The model under review builds one solid part; all positions refer to its coordinate system, in mm. A direction names the side the tool comes from. Give positions to 0.01 mm unless a question says otherwise; leave off trailing zeros. Order: outer loops, then holes, each group sorted by start corner. A loop starts at its lowest first (then second) coordinate and runs counter-clockwise, first axis right, second up. Notation, with made-up numbers: (78, -9.5) - (121, -9.5) arc R18 ccw to (121, 6.5) - close; hole circle Ø11 at (-5.75, 60.25). An arc over 180 degrees is marked (long way). Use a Markdown table: item, result. Add a question column.
```python
from build123d import *

# Parameters (mm, degrees)
RESSALTO_EXTRUS_O1_DEPTH = 25
ESBO_O2_R                = 3.75
ESBO_O2_R_2              = 1.65
CORTE_EXTRUS_O1_DEPTH    = 140.936789771
FILETE1_R                = 12.5
RESSALTO_EXTRUS_O2_REACH = 137.379
RESSALTO_EXTRUS_O3_DEPTH = 25
ESBO_O3_R                = 1.340765279
ESBO_O3_R_2              = 1.395401155
CORTE_EXTRUS_O4_DEPTH    = 25
ESBO_O10_R               = 1.55
CORTE_EXTRUS_O5_DEPTH    = 3


with BuildPart() as part:
    # Esboço1 → Ressalto-extrusão1 (new body)
    with BuildSketch(Plane(origin=(0, 0, 0), x_dir=(1, 0, 0), z_dir=(0, 1, 0))):
        Polygon((-59.715709909, 31.339816021), (-59.715709909, -1.660183979), (4.819954225, -7.306322984), (9.819954225, -7.306322984), (74.355618358, -1.660183979), (74.355618358, 31.339816021), (69.59163611, 31.339816021), (69.59163611, 2.942120769), (9.819954225, -2.287223796), (4.819954225, -2.287223796), (-54.951727661, 2.942120769), (-54.951727661, 31.339816021), align=None)
    extrude(amount=RESSALTO_EXTRUS_O1_DEPTH)

    # Esboço2 → Corte-extrusão1 (cut, through all)
    with BuildSketch(Plane(origin=(74.355618358, 0, 0), x_dir=(0, 0, -1), z_dir=(1, 0, 0))):
        with Locations((15.839816021, 12.5)):
            Circle(ESBO_O2_R)
        with Locations((24.339816021, 12.5)):
            Circle(ESBO_O2_R_2)
        with Locations((15.839816021, 4)):
            Circle(ESBO_O2_R_2)
        with Locations((15.839816021, 21)):
            Circle(ESBO_O2_R_2)
        with Locations((7.339816021, 12.5)):
            Circle(ESBO_O2_R_2)
    extrude(amount=-CORTE_EXTRUS_O1_DEPTH, mode=Mode.SUBTRACT)

    # Filete1
    filete1_edges = [part.edges().sort_by_distance(p)[0] for p in [
        (-57.333718785, 25, -31.339816021),
        (-57.333718785, 0, -31.339816021),
        (71.973627234, 25, -31.339816021),
        (71.973627234, 0, -31.339816021),
    ]]
    fillet(filete1_edges, radius=FILETE1_R - 0.0001)  # a hair under: the kernel refuses the full size

    # Ressalto-extrusão2: up to this face of the body (flat: up to its plane)
    ressalto_extrus_o2_end = Plane(part.part.faces().sort_by_distance((-54.951727661, 0.378342318, -10.891018395))[0])
    # Esboço6 → Ressalto-extrusão2 (add, up to the picked face)
    with BuildSketch(Plane.ZY.offset(-69.59163611), mode=Mode.PRIVATE) as ressalto_extrus_o2_sk1:
        with BuildLine():
            ThreePointArc((-13.839816021, 0.059742768), (-3.239816021, 12.5), (-13.839816021, 24.940257232))
            Line((-13.839816021, 24.940257232), (-2.942120769, 25))
            Line((-2.942120769, 25), (-2.942120769, 0))
            Line((-2.942120769, 0), (-13.839816021, 0.059742768))
        make_face()
    ressalto_extrus_o2_tool1 = split(extrude(ressalto_extrus_o2_sk1.sketch, amount=RESSALTO_EXTRUS_O2_REACH, mode=Mode.PRIVATE), bisect_by=ressalto_extrus_o2_end, keep=Keep.BOTH, mode=Mode.PRIVATE)
    add(ressalto_extrus_o2_tool1.solids().sort_by(Axis((69.591636, 24.697413, -8.389473), (-1, 0, 0)))[0])

    # Esboço8 → Ressalto-extrusão3 (add)
    with BuildSketch(Plane(origin=(0, 0, 0), x_dir=(-1, 0, 0), z_dir=(0, -1, 0))):
        Polygon((54.951727661, 2.942120769), (-4.819954225, -2.287223796), (-9.819954225, -2.287223796), (-69.59163611, 2.942120769), align=None)
    extrude(amount=-RESSALTO_EXTRUS_O3_DEPTH)

    # Esboço3 → Corte-extrusão4 (cut)
    with BuildSketch(Plane.XY.offset(7.306322984)):
        with Locations((7.319954225, 7)):
            Circle(ESBO_O3_R)
        with Locations((7.319954225, 18)):
            Circle(ESBO_O3_R_2)
    extrude(amount=-CORTE_EXTRUS_O4_DEPTH, mode=Mode.SUBTRACT)

    # Esboço10 → Corte-extrusão5 (cut)
    with BuildSketch(Plane.XY.offset(-5.943677016)):
        with Locations(Location((7.319954225, 7, 0), (0, 0, 180))):
            Circle(ESBO_O10_R)
        with Locations(Location((7.319954225, 18, 0), (0, 0, 180))):
            Circle(ESBO_O10_R)
    extrude(amount=CORTE_EXTRUS_O5_DEPTH, mode=Mode.SUBTRACT)


solid = part.part
```
Q1. Draft analysis for pull direction Z (two halves, no side actions). For faces 3 (the cylindrical face through (-57.367, 3.759, -27.775)), 4 (the cylindrical face through (-57.3, 11.036, -8.101)), 5 (the flat face through (7, 12, 7.306)), state which applies: pulls with the +Z half, pulls with the -Z half, needs draft (parallel to the pull), parting line crosses it, or undercut.
Q2. Machinability: for faces 1 (the cylindrical face through (8.192, 12.251, -3.242)), 2 (the cylindrical face through (-57.3, 11.496, -23.03)), which of the approach directions +Z, -Z, +X, -X, +Y, -Y give a long, thin tool a straight path to every point of the face, cutting with its end or side? Answer none if there is none.
Q3. Wall thickness on probe 1 along X at (y, z) = (8.5, -18); probe 2 along X at (y, z) = (18, -3.55); probe 3 along Y at (x, z) = (-27, -10): over which ranges is each line inside the solid? List them lowest first.
Q4. We need section D-D (x = -33). Write out the cut boundary in (y, z).
Q5. We need section A-A (y = 21). Write out the cut boundary in (x, z).
Q6. We need section B-B (z = -24). Write out the cut boundary in (x, y).
Q7. Clearance check with flat-ended pins moving along their axes: P1, Ø0.9, axis at x = 8, y = 7, coming from the -Z side; P2, Ø8, axis at x = 5.5, y = 9.5, coming from the -Z side; P3, Ø3.5, axis at x = 8, y = 18, coming from the -Z side; P4, Ø10, axis at x = -34.5, y = 19, coming from the -Z side. State where each tip first meets the part, or that it passes through.
Q8. We need section C-C (y = 7). Write out the cut boundary in (x, z).
Here are the results:
| question | item | result |
|---|---|---|
| 1 | face 3 | pulls with the -Z half |
| 1 | face 4 | undercut |
| 1 | face 5 | pulls with the +Z half |
| 2 | face 1 | -Z |
| 2 | face 2 | +X, -X |
| 3 | probe 1 | -59.72 to -54.95, 69.59 to 74.36 |
| 3 | probe 2 | -59.72 to 5.77, 8.87 to 74.36 |
| 3 | probe 3 | 0.04 to 1.34, 23.66 to 24.96 |
| 4 | outline | (0, -2.94) - (0.06, -13.84) arc R12.6 cw to (24.94, -13.84) - (25, -2.94) - (25, 4) - (0, 4) - close |
| 5 | outline | (-59.72, -28.01) - (-54.95, -28.01) - (-54.95, -17.49) - (-59.72, -17.49) - close; (-59.72, -14.19) - (-54.95, -14.19) - (-54.95, -6.54) - (69.59, -6.54) - (69.59, -14.19) - (74.36, -14.19) - (74.36, 1.66) - (9.82, 7.31) - (4.82, 7.31) - (-59.72, 1.66) - close; (69.59, -28.01) - (74.36, -28.01) - (74.36, -17.49) - (69.59, -17.49) - close |
| 6 | outline | (-59.72, 1.11) - (-54.95, 1.11) - (-54.95, 10.89) - (-59.72, 10.89) - close; (-59.72, 14.11) - (-54.95, 14.11) - (-54.95, 23.89) - (-59.72, 23.89) - close; (69.59, 1.11) - (74.36, 1.11) - (74.36, 10.89) - (69.59, 10.89) - close; (69.59, 14.11) - (74.36, 14.11) - (74.36, 23.89) - (69.59, 23.89) - close |
| 7 | P1 | through |
| 7 | P2 | z = -5.36 |
| 7 | P3 | z = -5.53 |
| 7 | P4 | z = -10.69 |
| 8 | outline | (-59.72, -30.06) - (-54.95, -30.06) - (-54.95, -4.5) - (5.77, -4.5) - (5.77, -2.94) - (5.98, -2.94) - (5.98, 7.31) - (4.82, 7.31) - (-59.72, 1.66) - close; (8.66, -2.94) - (8.87, -2.94) - (8.87, -4.5) - (69.59, -4.5) - (69.59, -30.06) - (74.36, -30.06) - (74.36, 1.66) - (9.82, 7.31) - (8.66, 7.31) - close |
